from build123d import *

# Parameters (mm, degrees)
SKETCH_1_W               = 16
SKETCH_1_H               = 34
EXTRUDE_1_DEPTH          = 28.6
CUT_EXTRUDE_3_DEPTH      = 48.222452287
CUT_EXTRUDE_3_DEPTH_BACK = 48.222452287
SKETCH_5_W               = 28.6
SKETCH_5_H               = 11
CUT_EXTRUDE_4_DEPTH      = 2
CUT_EXTRUDE_5_DEPTH      = 48.222452287
CUT_EXTRUDE_5_DEPTH_BACK = 48.222452287
SKETCH_9_RX              = 4.963641166
SKETCH_9_RY              = 2.372005513
CUT_EXTRUDE_6_DEPTH      = 48.222452453
CUT_EXTRUDE_6_DEPTH_BACK = 48.222452453
SKETCH_9_3_RX            = 4.963641166
SKETCH_9_3_RY            = 2.372005513
SKETCH_9_3_RX_2          = 5.183271306


with BuildPart() as part:
    # 草图1 → 凸台-拉伸1 (new body)
    with BuildSketch(Plane.XY):
        with Locations((8, -17)):
            Rectangle(SKETCH_1_W, SKETCH_1_H)
    extrude(amount=EXTRUDE_1_DEPTH)

    # 草图2 → 切除-拉伸3 (cut, two sides: drawn at the far end of the back side and taken through both)
    with BuildSketch(Plane.XY.offset(28.6).offset(-CUT_EXTRUDE_3_DEPTH_BACK)):
        with BuildLine():
            Line((10.284151777, -34), (10.284151777, -29.7156247))
            ThreePointArc((10.284151777, -29.7156247), (10.533147893, -27.735236154), (11.264636476, -25.878124872))
            ThreePointArc((11.264636476, -25.878124872), (7.278286447, -17.137749258), (0.015079207, -23.4251154))
            Line((0.015079207, -23.4251154), (0, -34))
            Line((0, -34), (10.284151777, -34))
        make_face()
    extrude(amount=CUT_EXTRUDE_3_DEPTH + CUT_EXTRUDE_3_DEPTH_BACK, mode=Mode.SUBTRACT)


with BuildPart() as cut_extrude_3_piece_1:
    # of the separate pieces the step leaves, piece 1, a body of its own (cut_extrude_3_pieces)
    add(part.part.solids().sort_by_distance((0, 0, 0))[0])

    # 草图9 → 切除-拉伸5 (cut, two sides: drawn at the far end of the back side and taken through both)
    with BuildSketch(Plane.ZY.offset(-CUT_EXTRUDE_5_DEPTH_BACK)):
        with Locations(Location((4.109179501, -6.391876735), (0, 0, -90))):
            Ellipse(SKETCH_9_RX, SKETCH_9_RY)
    extrude(amount=CUT_EXTRUDE_5_DEPTH + CUT_EXTRUDE_5_DEPTH_BACK, mode=Mode.SUBTRACT)

    # 草图9<3> → 切除-拉伸6 (cut, two sides: drawn at the far end of the back side and taken through both)
    with BuildSketch(Plane.ZY.offset(-CUT_EXTRUDE_6_DEPTH_BACK)):
        with Locations(Location((4.109179501, -6.391876735), (0, 0, -90))):
            Ellipse(SKETCH_9_3_RX, SKETCH_9_3_RY)
        with Locations(Location((10.785935759, -6.172246595), (0, 0, 90))):
            Ellipse(SKETCH_9_3_RX_2, SKETCH_9_3_RY)
        with Locations(Location((19.131881081, -6.391876735), (0, 0, -90))):
            Ellipse(SKETCH_9_3_RX, SKETCH_9_3_RY)
        with Locations(Location((25.149746919, -6.391876735), (0, 0, -90))):
            Ellipse(SKETCH_9_3_RX, SKETCH_9_3_RY)
    extrude(amount=CUT_EXTRUDE_6_DEPTH + CUT_EXTRUDE_6_DEPTH_BACK, mode=Mode.SUBTRACT)


with BuildPart() as cut_extrude_3_piece_2:
    # of the separate pieces the step leaves, piece 2, a body of its own (cut_extrude_3_pieces)
    add(part.part.solids().sort_by_distance((0, -34, 0))[0])

    # 草图5 → 切除-拉伸4 (cut)
    with BuildSketch(Plane.ZY):
        with Locations((14.3, -28.5)):
            Rectangle(SKETCH_5_W, SKETCH_5_H)
    extrude(amount=-CUT_EXTRUDE_4_DEPTH, mode=Mode.SUBTRACT)


solid = cut_extrude_3_piece_1.part
Can you work these out from the model? Positions are in its coordinate system, mm. A direction names the side the tool comes from. Round coordinates to 2 decimals unless told otherwise and drop trailing zeros. One line per question, with ' | ' between items. Start each with the question number.
1) Suppose I cut it at B-B on x = 9.25. Count the separate pieces of the cut face and the enclosed holes in it, then the cut area to 3 significant figures.
2) If we mould it in two halves opening along Y, with no side actions, what happens to faces 1 (the flat face through (10, -13, 0)), 2 (the flat face through (13, -34, 14)), 3 (the cylindrical face through (10.526, -27.762, 14.1))? For each: released by +Y, released by -Y, zero draft, split by the parting line, or undercut.
3) On a 3-axis mill with a long thin cutter (end or side, diameter ignored), from which of +Z, -Z, +X, -X, +Y, -Y can I reach the whole of each face in a straight line? I mean faces 4 (the flat face through (10.284, -32, 14)), 5 (the flat face through (10, -13, 28.6)). Say none if no direction works.
4) I need wall thicknesses on line 1 (Z direction, x = 2.75, y = -7); line 2 (Y direction, x = 6, z = 7.75); line 3 (Y direction, x = 4, z = 5.25). Which ranges of each line are inside material? Lowest first, please. Write a range as [from, to].
5) I'm going to push flat-ended pins straight in: P1, Ø6, axis at y = -4.5, z = 9.5, coming from the +X side; P2, Ø2, axis at y = -32, z = 20.5, coming from the -X side. Where does each tip first touch, or does it pass through?
Return value:
1) separate pieces: 1 | enclosed holes: 4 | area: 364 mm2
2) face 1: zero draft | face 2: released by -Y | face 3: undercut
3) face 4: +Z, -Z, -X, -Y | face 5: +Z, +X, -X, +Y, -Y
4) line 1: z = [0, 1.76], [6.46, 8.44], [13.13, 16.78], [21.49, 22.8], [27.5, 28.6] | line 2: y = [-17, 0] | line 3: y = [-17.34, -10.74], [-2.04, 0]
5) P1: stops at x = 16 | P2: stops at x = 10.28
